```python
from build123d import *

# Parameters (mm, degrees)
SKETCH1_W           = 11
SKETCH1_H           = 30
SKETCH1_R           = 1.5
BOSS_EXTRUDE1_DEPTH = 10
SKETCH2_R           = 1.5
CUT_EXTRUDE1_DEPTH  = 34.481338086
FILLET1_R           = 4


with BuildPart() as part:
    # Sketch1 → Boss-Extrude1 (new body)
    with BuildSketch(Plane(origin=(0, 0, 0), x_dir=(1, 0, 0), z_dir=(0, 1, 0))):
        with Locations((5.5, 15)):
            Rectangle(SKETCH1_W, SKETCH1_H)
        with Locations(Location((6, 25, 0), (0, 0, 270))):
            Circle(SKETCH1_R, mode=Mode.SUBTRACT)
        with Locations(Location((6, 5, 0), (0, 0, 270))):
            Circle(SKETCH1_R, mode=Mode.SUBTRACT)
    extrude(amount=BOSS_EXTRUDE1_DEPTH)

    # Sketch2 → Cut-Extrude1 (cut, through all)
    with BuildSketch(Plane(origin=(11, 0, 0), x_dir=(0, 0, -1), z_dir=(1, 0, 0))):
        with Locations((11, 5.530453401)):
            Circle(SKETCH2_R)
        with Locations((21, 5.530453401)):
            Circle(SKETCH2_R)
    extrude(amount=-CUT_EXTRUDE1_DEPTH, mode=Mode.SUBTRACT)

    # Fillet1
    fillet1_edges = [part.edges().sort_by_distance(p)[0] for p in [
        (0, 5, -30),
        (11, 5, -30),
        (11, 5, 0),
        (0, 5, 0),
    ]]
    fillet(fillet1_edges, radius=FILLET1_R)


solid = part.part
```
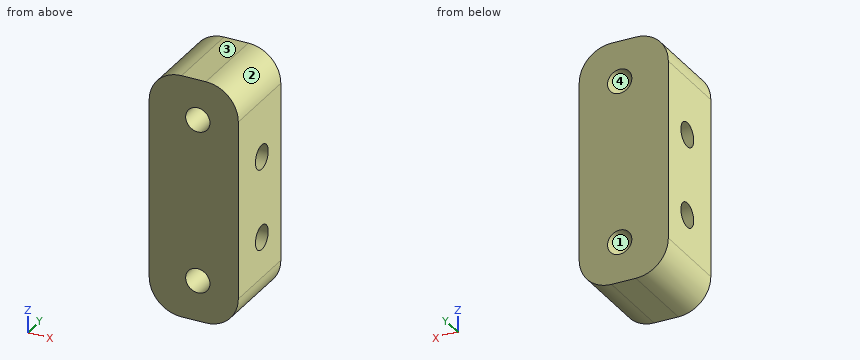
Build history of the part. All positions in model axes, mm. Face numbers are marked on the shaded views. Give positions to 0.01 mm unless a question says otherwise; leave off trailing zeros. Loops run counter-clockwise (first coordinate to the right, second up) from the corner with the lowest first, then second, coordinate; pieces in that order, holes last. Notation, with made-up numbers: (41.5, -18.75) - (75.5, -18.75) arc R30 ccw to (75.5, 16.25) - close; hole circle Ø11 at (7, 53.25). An arc over 180 degrees is marked (long way). Use a Markdown table: item, result.
(1) Band-saw the part on A-A (y = 6). Give the cut face in (x, z), and give its area (3 significant figures).
Taken from the geometry:
| item | result |
|---|---|
| outline | (0, -26) arc R4 ccw to (4, -30) - (7, -30) arc R4 ccw to (11, -26) - (11, -22.42) - (0, -22.42) - close; (0, -19.58) - (11, -19.58) - (11, -12.42) - (0, -12.42) - close; (0, -9.58) - (11, -9.58) - (11, -4) arc R4 ccw to (7, 0) - (4, 0) arc R4 ccw to (0, -4) - close; hole circle Ø3 at (6, -25); hole circle Ø3 at (6, -5) |
| area | 239 mm2 |
(2) Pull direction X, two halves, no side cores. Call the marked faces 1, 2, 3 and 4: +X half, -X half, draft (parallel to the pull), parting line (faces both ways), or undercut.
Taken from the geometry:
| item | result |
|---|---|
| face 1 | undercut |
| face 2 | +X half |
| face 3 | draft |
| face 4 | undercut |
(3) Band-saw the part on D-D (y = 7.5). Give the cut face in (x, z).
Taken from the geometry:
| item | result |
|---|---|
| outline | (0, -26) arc R4 ccw to (4, -30) - (7, -30) arc R4 ccw to (11, -26) - (11, -4) arc R4 ccw to (7, 0) - (4, 0) arc R4 ccw to (0, -4) - close; hole circle Ø3 at (6, -25); hole circle Ø3 at (6, -5) |
(4) Band-saw the part on B-B (z = -21). Give the cut face in (x, y).
Taken from the geometry:
| item | result |
|---|---|
| outline | (0, 0) - (11, 0) - (11, 4.03) - (0, 4.03) - close; (0, 7.03) - (11, 7.03) - (11, 10) - (0, 10) - close |
(5) Wall check: line 1 along Y through (x, z) = (7.5, -21); line 2 along X through (y, z) = (4.25, -25); line 3 along Z through (x, y) = (6.5, 2.25). Give the ranges that are in metal, low to high.
Taken from the geometry:
| item | result |
|---|---|
| line 1 | 0 to 4.03, 7.03 to 10 |
| line 2 | 0 to 4.5, 7.5 to 11 |
| line 3 | -30 to -26.41, -23.59 to -6.41, -3.59 to 0 |
(6) Drop flat-ended pins along their axis: pin 1 Ø1.8 at (x, z) = (6, -5) entering from +Y; pin 2 Ø1.5 at (y, z) = (7, -21) entering from -X; pin 3 Ø1.5 at (x, y) = (9.5, 4) entering from -Z. Give the stop position or say it passes through.
Taken from the geometry:
| item | result |
|---|---|
| pin 1 | through |
| pin 2 | x = 0 |
| pin 3 | z = -29.6 |
(7) Band-saw the part on C-C (x = 6). Give the cut face in (y, z).
Taken from the geometry:
| item | result |
|---|---|
| outline | (0, -30) - (10, -30) - (10, -26.5) - (0, -26.5) - close; (0, -23.5) - (10, -23.5) - (10, -6.5) - (0, -6.5) - close; (0, -3.5) - (10, -3.5) - (10, 0) - (0, 0) - close; hole circle Ø3 at (5.53, -21); hole circle Ø3 at (5.53, -11) |
